```python
from build123d import *

# Parameters (mm, degrees)
SKETCH_1_W          = 20.2
SKETCH_1_H          = 25
SKETCH_1_R          = 1.6
EXTRUDE_1_DEPTH     = 3.8
SKETCH_2_W          = 25
SKETCH_2_H          = 6
EXTRUDE_2_DEPTH     = 3.8
SKETCH_3_W          = 25
SKETCH_3_H          = 6
EXTRUDE_3_DEPTH     = 3.8
SKETCH_4_W          = 8
SKETCH_4_H          = 6
EXTRUDE_4_DEPTH     = 12
SKETCH_5_W          = 4.3
SKETCH_5_H          = 6
EXTRUDE_5_DEPTH     = 6
SKETCH_6_W          = 4.3
SKETCH_6_H          = 14
EXTRUDE_6_DEPTH     = 2
SKETCH_7_W          = 20.2
SKETCH_7_H          = 3.8
EXTRUDE_7_DEPTH     = 5
SKETCH_8_W          = 10
SKETCH_8_H          = 6
EXTRUDE_8_DEPTH     = 9
SKETCH_9_R          = 1.55
CUT_EXTRUDE_1_DEPTH = 3
SKETCH_10_R         = 1.05
CUT_EXTRUDE_2_DEPTH = 3
SKETCH_11_W         = 9
SKETCH_11_H         = 6
EXTRUDE_9_DEPTH     = 8
SKETCH_12_R         = 1.05
CUT_EXTRUDE_3_DEPTH = 48.885279575
CHAMFER_1_SIZE      = 2
SKETCH_13_R         = 1.55
CUT_EXTRUDE_4_DEPTH = 3
SKETCH_14_W         = 4.3
SKETCH_14_H         = 2
EXTRUDE_10_DEPTH    = 5
SKETCH_15_W         = 4.3
SKETCH_15_H         = 1
SKETCH_15_W_2       = 7.7
SKETCH_15_H_2       = 1.5
CUT_EXTRUDE_5_DEPTH = 10


with BuildPart() as part:
    # 草图1 → 凸台-拉伸1 (new body)
    with BuildSketch(Plane(origin=(0, 0, 0), x_dir=(1, 0, 0), z_dir=(0, 1, 0))):
        with Locations((10.1, 12.5)):
            Rectangle(SKETCH_1_W, SKETCH_1_H)
        with Locations(Location((2.6, 4.5, 0), (0, 0, 90))):
            Circle(SKETCH_1_R, mode=Mode.SUBTRACT)
        with Locations(Location((17.6, 4.5, 0), (0, 0, 90))):
            Circle(SKETCH_1_R, mode=Mode.SUBTRACT)
        with Locations(Location((17.6, 20.5, 0), (0, 0, 90))):
            Circle(SKETCH_1_R, mode=Mode.SUBTRACT)
        with Locations(Location((2.6, 20.5, 0), (0, 0, 90))):
            Circle(SKETCH_1_R, mode=Mode.SUBTRACT)
    extrude(amount=EXTRUDE_1_DEPTH)

    # 草图2 → 凸台-拉伸2 (add)
    with BuildSketch(Plane(origin=(20.2, 0, 0), x_dir=(0, 0, -1), z_dir=(1, 0, 0))):
        with Locations((12.5, 0.8)):
            Rectangle(SKETCH_2_W, SKETCH_2_H)
    extrude(amount=EXTRUDE_2_DEPTH)

    # 草图3 → 凸台-拉伸3 (add)
    with BuildSketch(Plane.ZY):
        with Locations((-12.5, 0.8)):
            Rectangle(SKETCH_3_W, SKETCH_3_H)
    extrude(amount=EXTRUDE_3_DEPTH)

    # 草图4 → 凸台-拉伸4 (add)
    with BuildSketch(Plane(origin=(24, 0, 0), x_dir=(0, 0, -1), z_dir=(1, 0, 0))):
        with Locations((21, 0.8)):
            Rectangle(SKETCH_4_W, SKETCH_4_H)
    extrude(amount=EXTRUDE_4_DEPTH)

    # 草图5 → 凸台-拉伸5 (add)
    with BuildSketch(Plane(origin=(0, 0, -25), x_dir=(-1, 0, 0), z_dir=(0, 0, -1))):
        with Locations((-33.85, 0.8)):
            Rectangle(SKETCH_5_W, SKETCH_5_H)
    extrude(amount=EXTRUDE_5_DEPTH)

    # 草图6 → 凸台-拉伸6 (add)
    with BuildSketch(Plane(origin=(0, -2.2, 0), x_dir=(-1, 0, 0), z_dir=(0, -1, 0))):
        with Locations((-33.85, 24)):
            Rectangle(SKETCH_6_W, SKETCH_6_H)
    extrude(amount=EXTRUDE_6_DEPTH)

    # 草图7 → 凸台-拉伸7 (add)
    with BuildSketch(Plane(origin=(0, 0, -25), x_dir=(-1, 0, 0), z_dir=(0, 0, -1))):
        Polygon((-20.2, 0), (-20.2, 3.8), (-24, 3.8), (-24, -2.2), (-20.2, -2.2), align=None)
        with Locations((-10.1, 1.9)):
            Rectangle(SKETCH_7_W, SKETCH_7_H)
        Polygon((3.8, -2.2), (3.8, 3.8), (0, 3.8), (0, 0), (0, -2.2), align=None)
    extrude(amount=EXTRUDE_7_DEPTH)

    # 草图8 → 凸台-拉伸8 (add)
    with BuildSketch(Plane.ZY.offset(3.8)):
        with Locations((-25, 0.8)):
            Rectangle(SKETCH_8_W, SKETCH_8_H)
    extrude(amount=EXTRUDE_8_DEPTH)

    # 草图9 → 切除-拉伸1 (cut)
    with BuildSketch(Plane(origin=(0, 3.8, 0), x_dir=(1, 0, 0), z_dir=(0, 1, 0))):
        with Locations(Location((-7.9, 26.5, 0), (0, 0, 270))):
            Circle(SKETCH_9_R)
        with Locations(Location((28.1, 19.5, 0), (0, 0, 270))):
            Circle(SKETCH_9_R)
    extrude(amount=-CUT_EXTRUDE_1_DEPTH, mode=Mode.SUBTRACT)

    # 草图10 → 切除-拉伸2 (cut)
    with BuildSketch(Plane(origin=(0, 0.8, 0), x_dir=(1, 0, 0), z_dir=(0, 1, 0))):
        with Locations(Location((-7.9, 26.5, 0), (0, 0, 270))):
            Circle(SKETCH_10_R)
        with Locations(Location((28.1, 19.5, 0), (0, 0, 270))):
            Circle(SKETCH_10_R)
    extrude(amount=-CUT_EXTRUDE_2_DEPTH, mode=Mode.SUBTRACT)

    # 草图11 → 凸台-拉伸9 (add)
    with BuildSketch(Plane.XY.offset(-20)):
        with Locations((-8.3, 0.8)):
            Rectangle(SKETCH_11_W, SKETCH_11_H)
    extrude(amount=EXTRUDE_9_DEPTH)

    # 草图12 → 切除-拉伸3 (cut, through all)
    with BuildSketch(Plane(origin=(0, -2.2, 0), x_dir=(-1, 0, 0), z_dir=(0, -1, 0))):
        with Locations(Location((6.9, 16.5, 0), (0, 0, 90))):
            Circle(SKETCH_12_R)
    extrude(amount=-CUT_EXTRUDE_3_DEPTH, mode=Mode.SUBTRACT)

    # 倒角1
    chamfer_1_edges = [part.edges().sort_by_distance(p)[0] for p in [
        (17.6, 3.8, -18.9),
        (2.6, 3.8, -18.9),
    ]]
    chamfer(chamfer_1_edges, length=CHAMFER_1_SIZE)

    # 草图13 → 切除-拉伸4 (cut)
    with BuildSketch(Plane(origin=(0, 3.8, 0), x_dir=(1, 0, 0), z_dir=(0, 1, 0))):
        with Locations(Location((-6.9, 16.5, 0), (0, 0, 270))):
            Circle(SKETCH_13_R)
    extrude(amount=-CUT_EXTRUDE_4_DEPTH, mode=Mode.SUBTRACT)

    # 草图14 → 凸台-拉伸10 (add)
    with BuildSketch(Plane.XY.offset(-17)):
        Polygon((24, 3.8), (24, -2.2), (31.7, -2.2), (36, -2.2), (36, 3.8), align=None)
        with Locations((33.85, -3.2)):
            Rectangle(SKETCH_14_W, SKETCH_14_H)
    extrude(amount=EXTRUDE_10_DEPTH)

    # 草图15 → 切除-拉伸5 (cut)
    with BuildSketch(Plane(origin=(0, 3.8, 0), x_dir=(1, 0, 0), z_dir=(0, 1, 0))):
        with Locations((33.85, 30.5)):
            Rectangle(SKETCH_15_W, SKETCH_15_H)
        with Locations((27.85, 24.25)):
            Rectangle(SKETCH_15_W_2, SKETCH_15_H_2)
    extrude(amount=-CUT_EXTRUDE_5_DEPTH, mode=Mode.SUBTRACT)


solid = part.part
```
Verification items for the finished model (mm, model axes). A direction names the side the tool comes from. Give positions to 0.01 mm unless a question says otherwise; leave off trailing zeros. Order: outer loops, then holes, each group sorted by start corner. A loop starts at its lowest first (then second) coordinate and runs counter-clockwise, first axis right, second up. Notation, with made-up numbers: (17.25, 77) -> (25.25, 77) arc R11 cw to (25.25, 97) -> close; hole circle Ø2 at (-39, 80). An arc over 180 degrees is marked (long way). Use a Markdown table: item, result.
1) Section check D-D, the plane z = -13.5. Record the boundary of the cut face in (x, y).
Results:
| item | result |
|---|---|
| outline | (-12.8, -2.2) -> (0, -2.2) -> (0, 0) -> (20.2, 0) -> (20.2, -2.2) -> (31.7, -2.2) -> (31.7, -4.2) -> (36, -4.2) -> (36, 3.8) -> (-12.8, 3.8) -> close |
2) Depth check by flat-ended pin: pin 1 Ø1.8 at (y, z) = (0, -8) entering from +X; pin 2 Ø1 at (x, z) = (10, -9.5) entering from -Y; pin 3 Ø10 at (x, z) = (-8.5, -7.5) entering from -Y. Enter the tip coordinate at first touch or a pass-through.
Results:
| item | result |
|---|---|
| pin 1 | x = 24 |
| pin 2 | y = 0 |
| pin 3 | y = -2.2 |
3) Tool access check on faces 1 (the flat face through (25, -2.2, -15)), 2 (the flat face through (-9, 0.8, -26)), 3 (the flat face through (28, 1, -23.5)). Record the directions out of +Z, -Z, +X, -X, +Y, -Y that give a thin tool (end or side, any length) a straight path to the whole face; none if there is none.
Results:
| item | result |
|---|---|
| face 1 | +Z, -Z, -X, -Y |
| face 2 | +Y |
| face 3 | -Z, +Y, -Y |
4) Section check B-B, the plane z = -10.25. Record the boundary of the cut face in (x, y).
Results:
| item | result |
|---|---|
| outline | (-3.8, -2.2) -> (0, -2.2) -> (0, 0) -> (20.2, 0) -> (20.2, -2.2) -> (24, -2.2) -> (24, 3.8) -> (-3.8, 3.8) -> close |
5) Section check A-A, the plane x = 28.1. Record the boundary of the cut face in (y, z).
Results:
| item | result |
|---|---|
| outline | (-2.2, -23.5) -> (3.8, -23.5) -> (3.8, -21.05) -> (0.8, -21.05) -> (0.8, -20.55) -> (-2.2, -20.55) -> close; (-2.2, -18.45) -> (0.8, -18.45) -> (0.8, -17.95) -> (3.8, -17.95) -> (3.8, -12) -> (-2.2, -12) -> close |
6) Mould release check, pull along X, two halves, no side actions. Record for faces 4 (the flat face through (30, 1, -12)), 5 (the flat face through (-3.8, 1, -6)), 6 (the flat face through (10, 0, -15)): pulls with the +X half, pulls with the -X half, needs draft (parallel to the pull), parting line crosses it, or undercut.
Results:
| item | result |
|---|---|
| face 4 | needs draft |
| face 5 | pulls with the -X half |
| face 6 | undercut |
7) Material ranges on probe 1 along Z at (x, y) = (17.6, 0.7); probe 2 along X at (y, z) = (-0.5, -16.5); probe 3 along X at (y, z) = (-0.75, -24.25), recorded low to high.
Results:
| item | result |
|---|---|
| probe 1 | -30 to -22.1, -18.9 to -6.1, -2.9 to 0 |
| probe 2 | -12.8 to -7.95, -5.85 to 0, 20.2 to 36 |
| probe 3 | -12.8 to 0, 20.2 to 24, 31.7 to 36 |
8) Section check C-C, the plane z = -5. Record the boundary of the cut face in (x, y), then the cut area to 3 significant figures.
Results:
| item | result |
|---|---|
| outline | (-3.8, -2.2) -> (0, -2.2) -> (0, 0) -> (1.08, 0) -> (1.08, 3.8) -> (-3.8, 3.8) -> close; (4.12, 0) -> (16.08, 0) -> (16.08, 3.8) -> (4.12, 3.8) -> close; (19.12, 0) -> (20.2, 0) -> (20.2, -2.2) -> (24, -2.2) -> (24, 3.8) -> (19.12, 3.8) -> close |
| area | 99.3 mm² |
